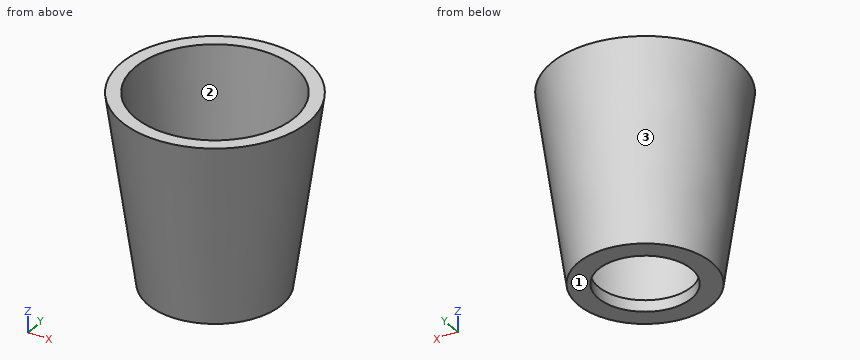
from build123d import *

# Parameters (mm, degrees)
SKETCH2_R           = 52.927862015
BOSS_EXTRUDE2_DEPTH = 150
BOSS_EXTRUDE2_DRAFT = -8
SKETCH6_R           = 36.849119173
CUT_EXTRUDE2_DEPTH  = 130
SKETCH8_R           = 63.168740943
CUT_EXTRUDE4_DEPTH  = 141
CUT_EXTRUDE4_DRAFT  = -5


with BuildPart() as part:
    # Sketch2 → Boss-Extrude2 (with draft: the straight prism first)
    with BuildSketch(Plane.XY):
        Circle(SKETCH2_R)
    extrude(amount=BOSS_EXTRUDE2_DEPTH)
    # Boss-Extrude2: the draft: its side faces are tilted about the plane it starts from
    boss_extrude2_sides = [part.faces().sort_by_distance(p)[0] for p in [
        (-52.927862015, 0, 75),
    ]]
    draft(boss_extrude2_sides, Plane.XY, BOSS_EXTRUDE2_DRAFT)

    # Sketch6 → Cut-Extrude2 (cut)
    with BuildSketch(Plane(origin=(0, 0, 0), x_dir=(-1, 0, 0), z_dir=(0, 0, -1))):
        Circle(SKETCH6_R)
    extrude(amount=-CUT_EXTRUDE2_DEPTH, mode=Mode.SUBTRACT)


with BuildPart() as cut_extrude4_tool:
    # Sketch8 → Cut-Extrude4 (with draft: the straight prism first)
    with BuildSketch(Plane.XY.offset(150)):
        Circle(SKETCH8_R)
    extrude(amount=-CUT_EXTRUDE4_DEPTH)
    # Cut-Extrude4: the draft: its side faces are tilted about the plane it starts from
    cut_extrude4_sides = [cut_extrude4_tool.faces().sort_by_distance(p)[0] for p in [
        (-63.168740943, 0, 79.5),
    ]]
    draft(cut_extrude4_sides, Plane.XY.offset(150), CUT_EXTRUDE4_DRAFT)


with BuildPart() as part_1:
    add(part.part)

    # Cut-Extrude4: cut by cut_extrude4_tool
    add(cut_extrude4_tool.part, mode=Mode.SUBTRACT)


solid = part_1.part
Geometry: final body of the model. Coordinates: model frame, mm. Face numbers are marked on the shaded views. Give positions to 0.01 mm unless a question says otherwise; leave off trailing zeros. Write each loop counter-clockwise with the first axis right and the second up, starting at its lowest first coordinate (ties: lowest second). Pieces come first, ordered by that corner, then holes.
(1) Cut plane C-C, the plane z = 83. Return loops of the section in (x, y), then the cut area to 3 significant figures.
(2) Cut plane D-D, the plane z = 24.5. Return loops of the section in (x, y), then the cut area to 3 significant figures.
(3) Mould query, pull axis X, two halves, no side actions, for the marked faces 1, 2 and 3. Classes: released by +X, released by -X, zero draft, split by the parting line, or undercut.
(4) First-contact query: P1, Ø4, axis at x = 25, z = 71, coming from the -Y side; P2, Ø6, axis at x = 6.5, z = 41, coming from the +Y side; P3, Ø5, axis at y = -24.5, z = 101.5, coming from the +X side. Flat tips, straight axial feed; report the tip coordinate or a pass-through.
(5) Cut plane A-A, the plane x = 0. Return loops of the section in (y, z).
(6) Ray query, line 1 (Z direction, x = 37, y = 14.5); line 2 (Y direction, x = -4.5, z = 75); line 3 (X direction, y = 25.5, z = 114). Return the intervals inside material, ascending.
Values follow:
1. outline: circle Ø129.19 at (0, 0); hole circle Ø114.61 at (0, 0)
1. area: 2,790 mm2
2. outline: circle Ø112.74 at (0, 0); hole circle Ø104.38 at (0, 0)
2. area: 1,430 mm2
3. face 1: zero draft
3. face 2: undercut
3. face 3: split by the parting line
4. P1: stops at y = -58.61
4. P2: stops at y = 58.84
4. P3: stops at x = 63.57
5. outline: (-74.01, 150) - (-52.93, 0) - (-36.85, 0) - (-36.85, 9) - (-50.83, 9) - (-63.17, 150) - close; (36.85, 0) - (52.93, 0) - (74.01, 150) - (63.17, 150) - (50.83, 9) - (36.85, 9) - close
6. line 1: z = 0 to 9
6. line 2: y = -63.31 to -56.43, 56.43 to 63.31
6. line 3: x = -64.06 to -54.33, 54.33 to 64.06
